Autodesk Inventor part; units mm, degrees
ref_plane "Work Plane1" through (-20, 0, 0) normal (0, 0, 1) x (1, 0, 0)
ref_plane "YZ Plane" through (0, 0, 0) normal (1, 0, 0) x (0, 1, 0)
ref_plane "XZ Plane" through (0, 0, 0) normal (0, 1, 0) x (-1, 0, 0)
sketch "Sketch1" plane through (0, 0, 0) normal (0, 1, 0) x (-1, 0, 0)
  line L0 (-20, -10) -> (20, -10)
  line L1 (20, -10) -> (20, 10)
  line L2 (20, 10) -> (-20, 10)
  line L3 (-20, 10) -> (-20, -10)
  line L4 (-20, -10) -> (20, 10) construction
  line L5 (20, -10) -> (-20, 10) construction
  point P0 (0, 0)
  dimension "d0" = 40
  dimension "d1" = 20
extrude "Extrusion1" add sketch "Sketch1" along normal blind 8
ref_plane "Work Plane1" through (-20, 0, 0) normal (0, 0, 1) x (1, 0, 0)
sketch "Sketch3" plane through (-20, 0, 0) normal (0, 0, 1) x (1, 0, 0)
  line L0 (0, 8) -> (40, 8)
  line L1 (40, 8) -> (30, 8)
  circle A0 centre (20, 8) radius 3.75
  line L2 (0, 0) -> (40, 0)
  line L3 (20, 8) -> (20, 10)
  line L4 (20, 10) -> (16.8279, 10)
  line L5 (20, 10) -> (23.1721, 10)
  line L6 (20, 8) -> (20, 2.75)
  point P0 (20, 0)
  point P1 (20, 4.25)
  dimension "d12" = 10
  dimension "d13" = 7.5
  dimension "d14" = 8
  dimension "d15" = 20
  dimension "d16" = 2
  dimension "d17" = 5.25
revolve "Revolution3" cut sketch "Sketch3" angle 360 about axis through (0, 8, 0) along (0, 1, 0) picked at (21.3217, 5.8965) contours L3 L5 A0 L0 | L0 A0 L6
fillet "Fillet2" radius 1 1 edges at (-3.75, 8, 0)
pattern_of_one "Rectangular Pattern2"
sketch "Sketch4" plane through (0, 8, 0) normal (0, 1, 0) x (1, 0, 0)
  line L0 (-20, 10) -> (-20, -10)
  line L1 (-20, 0) -> (-15, 0)
  line L2 (20, -10) -> (20, 10)
  line L3 (20, 0) -> (15, 0)
  circle A0 centre (-15, 0) radius 3
  circle A1 centre (15, 0) radius 3
  point P0 (0, 0)
  dimension "d33" = 5
  dimension "d34" = 5
  dimension "d35" = 6
  dimension "d36" = 6
extrude "Extrusion2" cut sketch "Sketch4" against normal blind 10
fillet "Fillet3" radius 3 4 edges at (0, 8, 10) (0, 8, -10) (-20, 8, 0) (20, 8, 0)
fillet "Fillet4" radius 3 4 edges at (0, 0, 10) (-20, 0, 0) (20, 0, 0) (0, 0, -10)
properties part number "TestBearingPad"
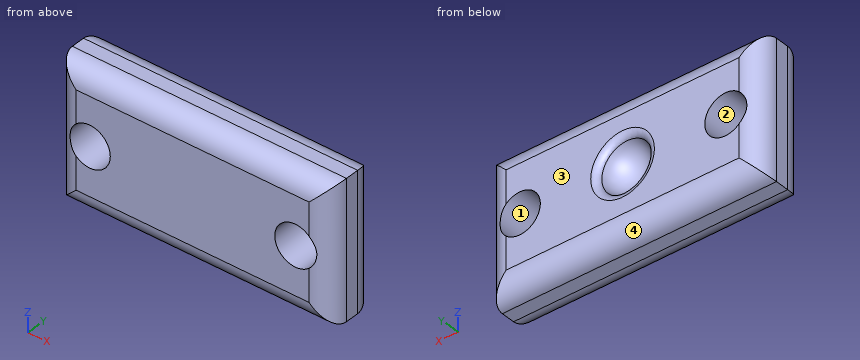
Work out the finished part from the listing and answer in its coordinate system (mm). Face numbers are marked on the shaded views. Give positions to 0.01 mm unless a question says otherwise; leave off trailing zeros. Order: outer loops, then holes, each group sorted by start corner. A loop starts at its lowest first (then second) coordinate and runs counter-clockwise, first axis right, second up. Notation, with made-up numbers: (-20, 42.25) - (-3, 42.25) arc R29 cw to (-3, 69.25) - close; hole circle Ø4 at (-10, 77.25). An arc over 180 degrees is marked (long way). Answer as CSV lines item,"result". Start each with the question number.
Q1. The part is cut by section C-C (z = 8.75). Write down the section's boundary in (x, y).
Q2. Find the intervals of material crossed by L1, parallel to Z at x = 15, y = 4.25; L2, parallel to X at y = 0.75, z = -1.5; L3, parallel to Z at x = 15.5, y = 0.5, in increasing order. Write a range as [from, to].
Q3. The mould has two halves that part along Z. Classify the marked faces 1, 2, 3 and 4: +Z half, -Z half, draft (parallel to the pull), parting line (faces both ways), or undercut.
Q4. The part is cut by section A-A (x = -15). Write down the section's boundary in (y, z), then the cut area to 3 significant figures.
Q5. The part is cut by section D-D (y = 2.5). Write down the section's boundary in (x, z), then the cut area to 3 significant figures.
Q6. Given pin 1 Ø5 at (x, z) = (-15, 0) entering from -Y; pin 2 Ø2 at (y, z) = (6.5, 4.5) entering from +X, each flat-ended and moving along its own axis, determine where each tip first touches the part or whether it passes through.
Q7. The part is cut by section B-B (y = 5.75). Write down the section's boundary in (x, z), then the cut area to 3 significant figures.
Check result:
1,outline,"(-20, 3) arc R3 ccw to (-18.75, 0.56) - (18.75, 0.56) arc R3 ccw to (20, 3) - (20, 5) arc R3 ccw to (18.75, 7.44) - (-18.75, 7.44) arc R3 ccw to (-20, 5) - close"
2,L1,"z = [-10, -3], [3, 10]"
2,L2,"x = [-18.98, -17.6], [-12.4, 12.4], [17.6, 18.98]"
2,L3,"z = [-8.66, -2.96], [2.96, 8.66]"
3,face 1,"undercut"
3,face 2,"undercut"
3,face 3,"draft"
3,face 4,"-Z half"
4,outline,"(0, -7) arc R3 ccw to (3, -10) - (5, -10) arc R3 ccw to (8, -7) - (8, -3) - (0, -3) - close; (0, 3) - (8, 3) - (8, 7) arc R3 ccw to (5, 10) - (3, 10) arc R3 ccw to (0, 7) - close"
4,area,"104 mm²"
5,outline,"(-19.96, -9.96) - (19.96, -9.96) - (19.96, 9.96) - (-19.96, 9.96) - close; hole circle Ø6 at (-15, 0); hole circle Ø6 at (15, 0)"
5,area,"738 mm²"
6,pin 1,"passes through"
6,pin 2,"stops at x = 19.96"
7,outline,"(-19.9, -9.9) - (19.9, -9.9) - (19.9, 9.9) - (-19.9, 9.9) - close; hole circle Ø6 at (-15, 0); hole circle Ø6 at (0, 0); hole circle Ø6 at (15, 0)"
7,area,"704 mm²"
